Input: part model. Units: mm. Frame: model coordinates. A direction names the side the tool comes from. Coordinates: 2 decimals unless noted, no trailing zeros. Write each loop counter-clockwise with the first axis right and the second up, starting at its lowest first coordinate (ties: lowest second). Pieces come first, ordered by that corner, then holes. Notation, with made-up numbers: (73.25, 69.5) - (80.25, 69.5) arc R33 ccw to (80.25, 107.5) - close; hole circle Ø10 at (23.5, 56). An arc over 180 degrees is marked (long way). Use a Markdown table: item, result. Add a question column.
Q1. Material intervals for probe 1 along X at (y, z) = (-6, 4.6); probe 2 along X at (y, z) = (4.5, 7.25); probe 3 along Z at (x, y) = (-22.5, 6.5), sorted ascending. Write a range as from..to.
Q2. Section query A-A (z = 4.6). Return the cut outline in (x, y).
Q3. Mould query, pull axis Z, two halves, no side actions, for faces 5 (the face through (0, 30, 17)), 6 (the face through (-21.531, 0.277, 6.463)), 7 (the face through (22, 0, 0)). Classes: released by +Z, released by -Z, zero draft, split by the parting line, or undercut.
Q4. Section query B-B (z = 11). Return the cut outline in (x, y), then the cut area to 3 significant figures.
Q5. Pin query (flat end, axial travel): P1, Ø4.5, axis at x = 22, z = 4.5, coming from the -Y side; P2, Ø11.5, axis at y = 5, z = 5.5, coming from the -X side; P3, Ø2.5, axis at x = -23.5, z = 5.5, coming from the +Y side. Return the tip coordinate at first contact, or that it passes through.
Q6. Section query C-C (x = 21.5). Return the cut outline in (y, z), then the cut area to 3 significant figures.
Q7. Set-up query: faces 1 (the face through (-22, 19.8, 8)), 2 (the face through (22, -19.8, 8)), 3 (the face through (-26.8, 0, 7)), 4 (the face through (18, 0, 7)). Return all of +Z, -Z, +X, -X, +Y, -Y with unobstructed straight access to the full face (end or side cutting, diameter ignored); none if empty.
Q8. Section query D-D (x = -22.5). Return the cut outline in (y, z), then the cut area to 3 significant figures.
from build123d import *

# Parameters (mm, degrees)
SKETCH2_W             = 53.6
SKETCH2_H             = 39.6
BOSS_EXTRUDE1_DEPTH   = 12
SKETCH3_W             = 70
SKETCH3_H             = 60
BOSS_EXTRUDE2_DEPTH   = 0.1
SKETCH4_R             = 2.1
CUT_EXTRUDE1_DEPTH    = 50.8
SKETCH5_W             = 36
SKETCH5_H             = 39.6
CUT_EXTRUDE2_DEPTH    = 12
CHAMFER1_SIZE         = 0.5
CHAMFER1_SIZE2        = 1.37373871
CHAMFER1_PART_2_SIZE  = 0.5
CHAMFER1_PART_2_SIZE2 = 1.37373871
BOSS_EXTRUDE3_DEPTH   = 60


with BuildPart() as part:
    # Sketch2 → Boss-Extrude1 (new body)
    with BuildSketch(Plane.XY):
        Rectangle(SKETCH2_W, SKETCH2_H)
    extrude(amount=BOSS_EXTRUDE1_DEPTH)

    # Sketch3 → Boss-Extrude2 (add)
    with BuildSketch(Plane.XY.offset(12)):
        Rectangle(SKETCH3_W, SKETCH3_H)
    extrude(amount=BOSS_EXTRUDE2_DEPTH)

    # Sketch4 → Cut-Extrude1 (cut, through all)
    with BuildSketch(Plane(origin=(0, 19.8, 0), x_dir=(1, 0, 0), z_dir=(0, 1, 0))):
        with Locations((22.5, -4.6)):
            Circle(SKETCH4_R)
        with Locations((-22.5, -4.6)):
            Circle(SKETCH4_R)
    extrude(amount=-CUT_EXTRUDE1_DEPTH, mode=Mode.SUBTRACT)

    # Sketch5 → Cut-Extrude2 (cut)
    with BuildSketch(Plane(origin=(0, 0, 0), x_dir=(-1, 0, 0), z_dir=(0, 0, -1))):
        Rectangle(SKETCH5_W, SKETCH5_H)
    extrude(amount=-CUT_EXTRUDE2_DEPTH, mode=Mode.SUBTRACT)

    # Chamfer1
    chamfer1_edges = [part.edges().sort_by_distance(p)[0] for p in [
        (-22.4, 19.8, 0),
        (-18, 0, 0),
        (-22.4, -19.8, 0),
        (-26.8, 0, 0),
    ]]
    chamfer1_side = [part.faces().sort_by_distance(p)[0] for p in [
        (-22.4, 0, 0),
    ]]
    chamfer(chamfer1_edges, length=CHAMFER1_SIZE, length2=CHAMFER1_SIZE2, reference=chamfer1_side[0])

    # Chamfer1 part 2
    chamfer1_part_2_edges = [part.edges().sort_by_distance(p)[0] for p in [
        (22.4, -19.8, 0),
        (18, 0, 0),
        (22.4, 19.8, 0),
        (26.8, 0, 0),
    ]]
    chamfer1_part_2_side = [part.faces().sort_by_distance(p)[0] for p in [
        (22.4, 0, 0),
    ]]
    chamfer(chamfer1_part_2_edges, length=CHAMFER1_PART_2_SIZE, length2=CHAMFER1_PART_2_SIZE2, reference=chamfer1_part_2_side[0])

    # Sketch6 → Boss-Extrude3 (add)
    with BuildSketch(Plane(origin=(0, 30, 0), x_dir=(1, 0, 0), z_dir=(0, 1, 0))):
        with BuildLine():
            Line((35, -12.1), (-35, -12.1))
            ThreePointArc((-35, -12.1), (0, -24.673593129), (35, -12.1))
        make_face()
    extrude(amount=-BOSS_EXTRUDE3_DEPTH)


solid = part.part
Values follow:
| question | item | result |
|---|---|---|
| 1 | probe 1 | -26.8..-24.6, -20.4..-18, 18..20.4, 24.6..26.8 |
| 1 | probe 2 | -26.8..-18, 18..26.8 |
| 1 | probe 3 | 0..2.5, 6.7..19.86 |
| 2 | outline | (-26.8, -19.8) - (-24.6, -19.8) - (-24.6, 19.8) - (-26.8, 19.8) - close; (-20.4, -19.8) - (-18, -19.8) - (-18, 19.8) - (-20.4, 19.8) - close; (18, -19.8) - (20.4, -19.8) - (20.4, 19.8) - (18, 19.8) - close; (24.6, -19.8) - (26.8, -19.8) - (26.8, 19.8) - (24.6, 19.8) - close |
| 3 | face 5 | zero draft |
| 3 | face 6 | undercut |
| 3 | face 7 | released by -Z |
| 4 | outline | (-26.8, -19.8) - (-18, -19.8) - (-18, 19.8) - (-26.8, 19.8) - close; (18, -19.8) - (26.8, -19.8) - (26.8, 19.8) - (18, 19.8) - close |
| 4 | area | 697 mm2 |
| 5 | P1 | y = -19.8 |
| 5 | P2 | x = -26.8 |
| 5 | P3 | y = 19.8 |
| 6 | outline | (-30, 12) - (-19.8, 12) - (-19.8, 6.45) - (19.8, 6.45) - (19.8, 12) - (30, 12) - (30, 20.3) - (-30, 20.3) - close; (-19.8, 1.37) - (-19.3, 0) - (19.3, 0) - (19.8, 1.37) - (19.8, 2.75) - (-19.8, 2.75) - close |
| 6 | area | 826 mm2 |
| 7 | face 1 | -Z, +X, -X, +Y |
| 7 | face 2 | -Z, +X, -X, -Y |
| 7 | face 3 | -Z, -X, +Y, -Y |
| 7 | face 4 | -Z, +Y, -Y |
| 8 | outline | (-30, 12) - (-19.8, 12) - (-19.8, 6.7) - (19.8, 6.7) - (19.8, 12) - (30, 12) - (30, 19.86) - (-30, 19.86) - close; (-19.8, 1.37) - (-19.3, 0) - (19.3, 0) - (19.8, 1.37) - (19.8, 2.5) - (-19.8, 2.5) - close |
| 8 | area | 780 mm2 |
